Design review of the part built by this model. Coordinates are the model's own, in mm. Face numbers are marked on the shaded views. A direction names the side the tool comes from. Coordinates: 2 decimals unless noted, no trailing zeros. Loops run counter-clockwise (first coordinate to the right, second up) from the corner with the lowest first, then second, coordinate; pieces in that order, holes last.
Q1. For P1, Ø14.5, axis at x = -1.5, y = -7, coming from the +Z side; P2, Ø4, axis at x = -6, z = 45.5, coming from the +Y side; P3, Ø3, axis at y = -1.5, z = 7.5, coming from the +X side, all flat-tipped, find the tip position at first contact; note any pin that passes through.
Q2. Wall thickness on probe 1 along X at (y, z) = (-18.05, 45.5); probe 2 along Z at (x, y) = (6, 15); probe 3 along Y at (x, z) = (12.5, 10): over which ranges is each line inside the solid? List them lowest first.
Q3. Draft analysis for pull direction Y (two halves, no side actions). For the marked faces 1, 2, 3 and 4, state which applies: released by +Y, released by -Y, zero draft, split by the parting line, or undercut.
Q4. Add section A-A on z = 45.5. Give the boundary of the cut face in (x, y), and give its area (4 significant figures).
Q5. Add section C-C on z = 39. Give the boundary of the cut face in (x, y), and give its area (4 significant figures).
Q6. Add section B-B on x = -6. Give the boundary of the cut face in (y, z), and give its area (3 significant figures).
Q7. Machinability: for the marked faces 5, 6 and 7, which of the approach directions +Z, -Z, +X, -X, +Y, -Y give a long, thin tool a straight path to every point of the face, cutting with its end or side? Answer none if there is none.
Q8. Add section D-D on y = 13. Give the boundary of the cut face in (x, z), and give its area (3 significant figures).
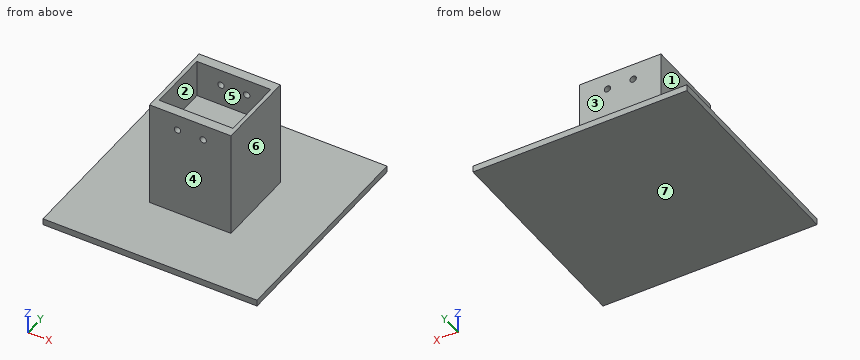
```python
from build123d import *

# Parameters (mm, degrees)
SKETCH1_W           = 100
SKETCH1_H           = 100
BOSS_EXTRUDE1_DEPTH = 3
SKETCH3_W           = 38
SKETCH3_H           = 38
BOSS_EXTRUDE2_DEPTH = 50
SKETCH5_W           = 34.5
SKETCH5_H           = 29
CUT_EXTRUDE1_DEPTH  = 17.5
SKETCH6_R           = 1.5
CUT_EXTRUDE2_DEPTH  = 50


with BuildPart() as part:
    # Sketch1 → Boss-Extrude1 (new body)
    with BuildSketch(Plane.XY):
        Rectangle(SKETCH1_W, SKETCH1_H)
    extrude(amount=BOSS_EXTRUDE1_DEPTH)

    # Sketch3 → Boss-Extrude2 (add)
    with BuildSketch(Plane.XY.offset(3)):
        Rectangle(SKETCH3_W, SKETCH3_H)
    extrude(amount=BOSS_EXTRUDE2_DEPTH)

    # Sketch5 → Cut-Extrude1 (cut)
    with BuildSketch(Plane.XY.offset(53)):
        Rectangle(SKETCH5_W, SKETCH5_H)
    extrude(amount=-CUT_EXTRUDE1_DEPTH, mode=Mode.SUBTRACT)

    # Sketch6 → Cut-Extrude2 (cut)
    with BuildSketch(Plane(origin=(0, 19, 0), x_dir=(1, 0, 0), z_dir=(0, 1, 0))):
        with Locations((6, -45.5)):
            Circle(SKETCH6_R)
        with Locations((-6, -45.5)):
            Circle(SKETCH6_R)
    extrude(amount=-CUT_EXTRUDE2_DEPTH, mode=Mode.SUBTRACT)


solid = part.part
```
Entries:
1. P1: stops at z = 35.5
1. P2: stops at y = 19
1. P3: stops at x = 19
2. probe 1: x = -19 to -7.5, -4.5 to 4.5, 7.5 to 19
2. probe 2: z = 0 to 44, 47 to 53
2. probe 3: y = -19 to 19
3. face 1: zero draft
3. face 2: undercut
3. face 3: released by +Y
3. face 4: released by -Y
4. outline: (-19, -19) - (-7.5, -19) - (-7.5, -14.5) - (-17.25, -14.5) - (-17.25, 14.5) - (-7.5, 14.5) - (-7.5, 19) - (-19, 19) - close; (-4.5, -19) - (4.5, -19) - (4.5, -14.5) - (-4.5, -14.5) - close; (-4.5, 14.5) - (4.5, 14.5) - (4.5, 19) - (-4.5, 19) - close; (7.5, -19) - (19, -19) - (19, 19) - (7.5, 19) - (7.5, 14.5) - (17.25, 14.5) - (17.25, -14.5) - (7.5, -14.5) - close
4. area: 389.5 mm2
5. outline: (-19, -19) - (19, -19) - (19, 19) - (-19, 19) - close; hole (-17.25, -14.5) - (17.25, -14.5) - (17.25, 14.5) - (-17.25, 14.5) - close
5. area: 443.5 mm2
6. outline: (-50, 0) - (50, 0) - (50, 3) - (19, 3) - (19, 44) - (14.5, 44) - (14.5, 35.5) - (-14.5, 35.5) - (-14.5, 44) - (-19, 44) - (-19, 3) - (-50, 3) - close; (-19, 47) - (-14.5, 47) - (-14.5, 53) - (-19, 53) - close; (14.5, 47) - (19, 47) - (19, 53) - (14.5, 53) - close
6. area: 1,670 mm2
7. face 5: +Z
7. face 6: +Z, +X, +Y, -Y
7. face 7: -Z, +X, -X, +Y, -Y
8. outline: (-50, 0) - (50, 0) - (50, 3) - (19, 3) - (19, 53) - (17.25, 53) - (17.25, 35.5) - (-17.25, 35.5) - (-17.25, 53) - (-19, 53) - (-19, 3) - (-50, 3) - close
8. area: 1,600 mm2
